```python
from build123d import *

# Parameters (mm, degrees)
F0_R     = 7
F0_R_2   = 2
F0_R_3   = 2.5
F0_R_4   = 5
F1_DEPTH = 9
F0_R_5   = 3.5
F2_DEPTH = 5


with BuildPart() as f1:
    # F0 (on Front) → F1 (new body)
    with BuildSketch(Plane.XZ):
        with BuildLine():
            ThreePointArc((-70, 10), (-67.071068, 2.928932), (-60, 0))
            Line((-60, 0), (60, 0))
            ThreePointArc((60, 0), (67.071068, 2.928932), (70, 10))
            Line((70, 10), (70, 96.972244))
            ThreePointArc((70, 96.972244), (69.57092, 99.870085), (68.320503, 102.519246))
            Line((68.320503, 102.519246), (32.968665, 155.547002))
            ThreePointArc((32.968665, 155.547002), (29.366742, 158.816746), (24.648162, 160))
            Line((24.648162, 160), (-24.648162, 160))
            ThreePointArc((-24.648162, 160), (-29.366742, 158.816746), (-32.968665, 155.547002))
            Line((-32.968665, 155.547002), (-68.320503, 102.519246))
            ThreePointArc((-68.320503, 102.519246), (-69.57092, 99.870085), (-70, 96.972244))
            Line((-70, 96.972244), (-70, 10))
        make_face()
        with Locations((-57.5, 10)):
            Circle(F0_R, mode=Mode.SUBTRACT)
        with Locations((-66, 31)):
            Circle(F0_R_2, mode=Mode.SUBTRACT)
        with Locations((-20, 10)):
            Circle(F0_R_3, mode=Mode.SUBTRACT)
        with Locations((-20, 31)):
            Circle(F0_R_3, mode=Mode.SUBTRACT)
        with Locations((-66, 50)):
            Circle(F0_R_2, mode=Mode.SUBTRACT)
        with Locations((-66, 69)):
            Circle(F0_R_2, mode=Mode.SUBTRACT)
        with Locations((-20, 50)):
            Circle(F0_R_3, mode=Mode.SUBTRACT)
        with Locations((-20, 69)):
            Circle(F0_R_3, mode=Mode.SUBTRACT)
        with Locations((0, 10)):
            Circle(F0_R, mode=Mode.SUBTRACT)
        with Locations((20, 10)):
            Circle(F0_R_3, mode=Mode.SUBTRACT)
        with Locations((20, 31)):
            Circle(F0_R_3, mode=Mode.SUBTRACT)
        with Locations((57.5, 10)):
            Circle(F0_R, mode=Mode.SUBTRACT)
        with Locations((66, 31)):
            Circle(F0_R_2, mode=Mode.SUBTRACT)
        with Locations((20, 50)):
            Circle(F0_R_3, mode=Mode.SUBTRACT)
        with Locations((20, 69)):
            Circle(F0_R_3, mode=Mode.SUBTRACT)
        with Locations((66, 50)):
            Circle(F0_R_2, mode=Mode.SUBTRACT)
        with Locations((66, 69)):
            Circle(F0_R_2, mode=Mode.SUBTRACT)
        with Locations((-57.5, 90)):
            Circle(F0_R_4, mode=Mode.SUBTRACT)
        with BuildLine():
            ThreePointArc((-19.264297, 92.610703), (-22.011126, 96.485049), (-17.5, 95))
            ThreePointArc((-17.5, 95), (-17.527831, 94.628008), (-17.610703, 94.264297))
            ThreePointArc((-17.610703, 94.264297), (-12.555978, 94.361967), (-10, 90))
            ThreePointArc((-10, 90), (-16.356192, 85.187439), (-19.264297, 92.610703))
        make_face(mode=Mode.SUBTRACT)
        with BuildLine():
            ThreePointArc((-17, 110), (-15.5, 111.5), (-14, 110))
            Line((-14, 110), (-14, 100))
            ThreePointArc((-14, 100), (-15.5, 98.5), (-17, 100))
            Line((-17, 100), (-17, 110))
        make_face(mode=Mode.SUBTRACT)
        with Locations((-20, 120.5)):
            Circle(F0_R_3, mode=Mode.SUBTRACT)
        with BuildLine():
            ThreePointArc((-17, 141), (-15.5, 142.5), (-14, 141))
            Line((-14, 141), (-14, 131))
            ThreePointArc((-14, 131), (-15.5, 129.5), (-17, 131))
            Line((-17, 131), (-17, 141))
        make_face(mode=Mode.SUBTRACT)
        with Locations((-20, 150)):
            Circle(F0_R_3, mode=Mode.SUBTRACT)
        with BuildLine():
            ThreePointArc((17.610703, 94.264297), (19.628008, 97.472169), (22.5, 95))
            ThreePointArc((22.5, 95), (21.485049, 92.988874), (19.264297, 92.610703))
            ThreePointArc((19.264297, 92.610703), (19.812561, 91.356192), (20, 90))
            ThreePointArc((20, 90), (10.638033, 87.555978), (17.610703, 94.264297))
        make_face(mode=Mode.SUBTRACT)
        with BuildLine():
            ThreePointArc((14, 110), (15.5, 111.5), (17, 110))
            Line((17, 110), (17, 100))
            ThreePointArc((17, 100), (15.5, 98.5), (14, 100))
            Line((14, 100), (14, 110))
        make_face(mode=Mode.SUBTRACT)
        with Locations((57.5, 90)):
            Circle(F0_R_4, mode=Mode.SUBTRACT)
        with BuildLine():
            ThreePointArc((-11, 125.5), (0, 136.5), (11, 125.5))
            Line((11, 125.5), (11, 115.5))
            ThreePointArc((11, 115.5), (0, 104.5), (-11, 115.5))
            Line((-11, 115.5), (-11, 125.5))
        make_face(mode=Mode.SUBTRACT)
        with BuildLine():
            ThreePointArc((14, 141), (15.5, 142.5), (17, 141))
            Line((17, 141), (17, 131))
            ThreePointArc((17, 131), (15.5, 129.5), (14, 131))
            Line((14, 131), (14, 141))
        make_face(mode=Mode.SUBTRACT)
        with Locations((20, 120.5)):
            Circle(F0_R_3, mode=Mode.SUBTRACT)
        with Locations((20, 150)):
            Circle(F0_R_3, mode=Mode.SUBTRACT)
    extrude(amount=F1_DEPTH)

    # F0 (on Front) → F2 (join)
    with BuildSketch(Plane.XZ):
        with Locations((-57.5, 90)):
            Circle(F0_R_4)
        with Locations((-57.5, 90)):
            Circle(F0_R_3, mode=Mode.SUBTRACT)
        with BuildLine():
            ThreePointArc((-17.610703, 94.264297), (-18.232233, 93.232233), (-19.264297, 92.610703))
            ThreePointArc((-19.264297, 92.610703), (-16.356192, 85.187439), (-10, 90))
            ThreePointArc((-10, 90), (-12.555978, 94.361967), (-17.610703, 94.264297))
        make_face()
        with Locations((-15, 90)):
            Circle(F0_R_3, mode=Mode.SUBTRACT)
        with BuildLine():
            ThreePointArc((19.264297, 92.610703), (18.232233, 93.232233), (17.610703, 94.264297))
            ThreePointArc((17.610703, 94.264297), (10.638033, 87.555978), (20, 90))
            ThreePointArc((20, 90), (19.812561, 91.356192), (19.264297, 92.610703))
        make_face()
        with Locations((15, 90)):
            Circle(F0_R_3, mode=Mode.SUBTRACT)
        with Locations((57.5, 90)):
            Circle(F0_R_4)
        with Locations((57.5, 90)):
            Circle(F0_R_3, mode=Mode.SUBTRACT)
        with Locations((57.5, 10)):
            Circle(F0_R)
        with Locations((57.5, 10)):
            Circle(F0_R_5, mode=Mode.SUBTRACT)
        with Locations((0, 10)):
            Circle(F0_R)
        with Locations((0, 10)):
            Circle(F0_R_5, mode=Mode.SUBTRACT)
        with Locations((-57.5, 10)):
            Circle(F0_R)
        with Locations((-57.5, 10)):
            Circle(F0_R_5, mode=Mode.SUBTRACT)
    extrude(amount=F2_DEPTH)


solid = f1.part
```
Geometry: final body of the model. Coordinates: model frame, mm. A direction names the side the tool comes from. Give positions to 0.01 mm unless a question says otherwise; leave off trailing zeros. Loops run counter-clockwise (first coordinate to the right, second up) from the corner with the lowest first, then second, coordinate; pieces in that order, holes last. Notation, with made-up numbers: (38, 79.5) -> (74, 79.5) arc R21 ccw to (74, 118.5) -> close; hole circle Ø8 at (29, 13.5). An arc over 180 degrees is marked (long way). Use one line per item in the form item = value.
Item 1: Section query A-A on x = 0. Output: boundary loops of the cut face in (y, z).
A:
outline = (-9, 0) -> (0, 0) -> (0, 6.5) -> (-5, 6.5) -> (-5, 3) -> (-9, 3) -> close; (-9, 17) -> (-5, 17) -> (-5, 13.5) -> (0, 13.5) -> (0, 104.5) -> (-9, 104.5) -> close; (-9, 136.5) -> (0, 136.5) -> (0, 160) -> (-9, 160) -> close
Item 2: Section query C-C on x = 35. Output: boundary loops of the cut face in (y, z), and give its area (3 significant figures).
A:
outline = (-9, 0) -> (0, 0) -> (0, 152.5) -> (-9, 152.5) -> close
area = 1,370 mm^2
Item 3: Draft query along Z for faces 1 (the face through (-67.15, -4.44, 3.01)), 2 (the face through (50.892, -4.437, 128.662)), 3 (the face through (-65.077, -4.437, 48.226)), 4 (the face through (-0.2, -4.4, 136.5)). Return one class per face: pulls with the +Z half, pulls with the -Z half, needs draft (parallel to the pull), parting line crosses it, or undercut.
A:
face_1 = pulls with the -Z half
face_2 = pulls with the +Z half
face_3 = undercut
face_4 = undercut
Item 4: Line query: probe 1 along Z at (x, y) = (0, -7); probe 2 along X at (y, z) = (-8, 29.5); probe 3 along Z at (x, y) = (-56.5, -3.25). Output: solid intervals per line, ascending.
A:
probe_1 = 0 to 3, 17 to 104.5, 136.5 to 160
probe_2 = -70 to -67.32, -64.68 to -22, -18 to 18, 22 to 64.68, 67.32 to 70
probe_3 = 0 to 6.65, 13.35 to 87.71, 92.29 to 120.25
Item 5: Pin query (flat end, axial travel): P1, Ø12.5, axis at x = -57.5, z = 10, coming from the -Y side; P2, Ø3, axis at x = -57.5, z = 90, coming from the +Y side; P3, Ø2.5, axis at y = -3, z = 119, coming from the -X side; P4, Ø2.5, axis at y = -4, z = 106, coming from the +X side. Return the tip coordinate at first contact, or that it passes through.
A:
P1 = -5
P2 = through
P3 = -58.17
P4 = 66.83
Item 6: Access query for faces 5 (the face through (55, -5, 89)), 6 (the face through (17, -4, 136)), 7 (the face through (-69.56, -4.44, 99.91)). Directions: +Z, -Z, +X, -X, +Y, -Y. A direction counts if a zero-diameter tool reaches every point of the face in a straight line with its end or side. Return the directions, or none.
A:
face_5 = -Y
face_6 = +Y, -Y
face_7 = +Z, -X, +Y, -Y
Item 7: Section query B-B on y = -7.5. Give the number of separate pieces and of enclosed holes in the cut face, and give its area (3 significant figures).
A:
separate_pieces = 1
enclosed_holes = 30
area = 18,100 mm^2
